from build123d import *

# Parameters (mm, degrees)
SKETCH2_W           = 120
SKETCH2_H           = 20
BOSS_EXTRUDE1_DEPTH = 8
CUT_EXTRUDE1_DEPTH  = 40
SKETCH4_R           = 4
CUT_EXTRUDE2_DEPTH  = 10


with BuildPart() as part:
    # Sketch2 → Boss-Extrude1 (new body)
    with BuildSketch(Plane(origin=(0, 0, 0), x_dir=(1, 0, 0), z_dir=(0, 1, 0))):
        with Locations((60, 10)):
            Rectangle(SKETCH2_W, SKETCH2_H)
    extrude(amount=BOSS_EXTRUDE1_DEPTH)

    # Sketch3 → Cut-Extrude1 (cut)
    with BuildSketch(Plane(origin=(0, 8, 0), x_dir=(1, 0, 0), z_dir=(0, 1, 0))):
        Polygon((10, 0), (0, 20), (0, 0), align=None)
        Polygon((120, 0), (120, 20), (110, 0), align=None)
        Polygon((60, 12), (60, 20), (20, 20), (25, 12), align=None)
        Polygon((100, 20), (60, 20), (60, 12), (95, 12), align=None)
    extrude(amount=-CUT_EXTRUDE1_DEPTH, mode=Mode.SUBTRACT)

    # Sketch4 → Cut-Extrude2 (cut)
    with BuildSketch(Plane(origin=(0, 8, 0), x_dir=(1, 0, 0), z_dir=(0, 1, 0))):
        with Locations(Location((14, 13, 0), (0, 0, 270))):
            Circle(SKETCH4_R)
        with Locations(Location((53, 6, 0), (0, 0, 270))):
            Circle(SKETCH4_R)
        with Locations(Location((67, 6, 0), (0, 0, 270))):
            Circle(SKETCH4_R)
        with Locations(Location((106, 13, 0), (0, 0, 270))):
            Circle(SKETCH4_R)
    extrude(amount=-CUT_EXTRUDE2_DEPTH, mode=Mode.SUBTRACT)


solid = part.part
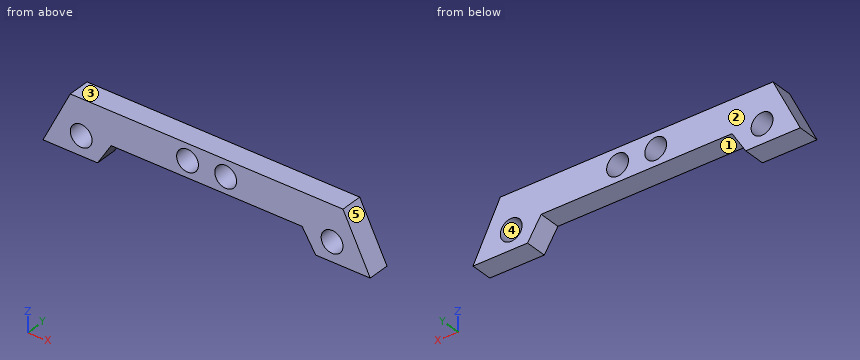
CAD build for the part. Positions are in the model's coordinates, mm. Face numbers are marked on the shaded views. A direction names the side the tool comes from. Round coordinates to 2 decimals unless told otherwise and drop trailing zeros. Order: outer loops, then holes, each group sorted by start corner. A loop starts at its lowest first (then second) coordinate and runs counter-clockwise, first axis right, second up. Notation, with made-up numbers: (71.5, 63) - (84.5, 63) arc R27 cw to (84.5, 96) - close; hole circle Ø4 at (53.25, 17). An arc over 180 degrees is marked (long way). Return JSON: item names as keys, results as strings.
(1) Cut at C-C (y = 1). Give the cut face in (x, z).
Answer key:
{"outline": "(0, -20) - (20, -20) - (25, -12) - (95, -12) - (100, -20) - (120, -20) - (110, 0) - (10, 0) - close; hole circle Ø8 at (14, -13); hole circle Ø8 at (53, -6); hole circle Ø8 at (67, -6); hole circle Ø8 at (106, -13)"}
(2) Tool access for the marked faces 1 and 2: list every direction of +Z, -Z, +X, -X, +Y, -Y with a clear straight run to the whole face (end or side of a thin tool).
Answer key:
{"face 1": "-Z, +Y, -Y", "face 2": "+Z, -Z, +X, -X, +Y"}
(3) Cut at B-B (x = 106). Give the cut face in (y, z).
Answer key:
{"outline": "(0, -20) - (8, -20) - (8, -17) - (0, -17) - close; (0, -9) - (8, -9) - (8, 0) - (0, 0) - close"}
(4) Pull direction X, two halves, no side cores. Call the marked faces 3, 4 and 5: +X half, -X half, draft (parallel to the pull), parting line (faces both ways), or undercut.
Answer key:
{"face 3": "draft", "face 4": "undercut", "face 5": "+X half"}
(5) Wall check: probe 1 along X at (y, z) = (6, -13) (3 decimals); probe 2 along X at (y, z) = (1.5, -6); probe 3 along X at (y, z) = (7, -2.75) (3 decimals). Give the ranges that are in metal, low to high. Write a range as from..to.
Answer key:
{"probe 1": "x = 3.5..10, 18..24.375, 95.625..102, 110..116.5", "probe 2": "x = 7..49, 57..63, 71..113", "probe 3": "x = 8.625..50.668, 55.332..64.668, 69.332..111.375"}
(6) Pin check, flat tips, straight feed: pin 1 Ø1.5 at (x, y) = (63, 5) entering from -Z; pin 2 Ø4 at (y, z) = (4.5, -7) entering from -X; pin 3 Ø2 at (y, z) = (6.5, -15.5) entering from +X. Stop position of each tip, or through.
Answer key:
{"pin 1": "stops at z = -12", "pin 2": "stops at x = 5.5", "pin 3": "stops at x = 118.25"}
(7) Cut at D-D (z = -18.25). Give the cut face in (x, y) (3 decimals).
Answer key:
{"outline": "(0.875, 0) - (21.094, 0) - (21.094, 8) - (0.875, 8) - close; (98.906, 0) - (119.125, 0) - (119.125, 8) - (98.906, 8) - close"}
(8) Cut at A-A (z = -6). Give the cut face in (x, y), then the cut area to 3 significant figures.
Answer key:
{"outline": "(7, 0) - (49, 0) - (49, 8) - (7, 8) - close; (57, 0) - (63, 0) - (63, 8) - (57, 8) - close; (71, 0) - (113, 0) - (113, 8) - (71, 8) - close", "area": "720 mm^2"}
